Input: part model. Units: mm. Frame: model coordinates. A direction names the side the tool comes from. Coordinates: 2 decimals unless noted, no trailing zeros. Loops run counter-clockwise (first coordinate to the right, second up) from the corner with the lowest first, then second, coordinate; pieces in that order, holes last.
(1) Section C-C, the plane y = 5.5. Return loops of the section in (x, z), then the cut area to 3 significant figures.
(2) Mould query, pull axis Z, two halves, no side actions, for faces 1 (the face through (43, 5, 80)), 2 (the face through (10, 5, 55)), 3 (the face through (13.01, 4.93, 97.15)). Classes: released by +Z, released by -Z, zero draft, split by the parting line, or undercut.
(3) Line query: L1, parallel to X at y = 27, z = 0; L2, parallel to X at y = 9, z = 38; L3, parallel to X at y = 24, z = -1. Output: solid intervals per line, ascending.
(4) Contact query for flat-ended pins moving along their axis: P1, Ø11, axis at y = 4.5, z = 47, coming from the -X side; P2, Ø3, axis at y = 21.5, z = 2, coming from the -X side; P3, Ø8, axis at x = 75.5, y = 19, coming from the -Z side. Output: stop coordinate, or through.
(5) Section B-B, the plane z = 0. Return loops of the section in (x, y), then the cut area to 3 significant figures.
(6) Section D-D, the plane z = 62. Return loops of the section in (x, y).
(7) Section A-A, the plane x = 47. Return loops of the section in (y, z), then the cut area to 3 significant figures.
(8) Set-up query: faces 4 (the face through (-19.524, 24.164, -4.336)), 5 (the face through (40, 10, 59)), 6 (the face through (70, 5, 55)). Return all of +Z, -Z, +X, -X, +Y, -Y with unobstructed straight access to the full face (end or side cutting, diameter ignored); none if empty.
```python
from build123d import *

# Parameters (mm, degrees)
SKETCH1_R           = 20
BOSS_EXTRUDE1_DEPTH = 40
SKETCH2_R           = 10
CUT_EXTRUDE1_DEPTH  = 49.989794856
SKETCH3_R           = 20
BOSS_EXTRUDE2_DEPTH = 30
SKETCH4_R           = 10
CUT_EXTRUDE2_DEPTH  = 107.301458127
SKETCH5_W           = 80
SKETCH5_H           = 10
BOSS_EXTRUDE3_DEPTH = 30
BOSS_EXTRUDE4_DEPTH = 10
BOSS_EXTRUDE5_DEPTH = 10


with BuildPart() as part:
    # Sketch1 → Boss-Extrude1 (new body)
    with BuildSketch(Plane(origin=(0, 0, 0), x_dir=(1, 0, 0), z_dir=(0, 1, 0))):
        with Locations(Location((0, 0, 0), (0, 0, 270))):
            Circle(SKETCH1_R)
    extrude(amount=BOSS_EXTRUDE1_DEPTH)

    # Sketch2 → Cut-Extrude1 (cut, through all)
    with BuildSketch(Plane(origin=(0, 40, 0), x_dir=(1, 0, 0), z_dir=(0, 1, 0))):
        with Locations(Location((0, 0, 0), (0, 0, 270))):
            Circle(SKETCH2_R)
    extrude(amount=-CUT_EXTRUDE1_DEPTH, mode=Mode.SUBTRACT)



with BuildPart() as body_2:
    # Sketch3 → Boss-Extrude2 (new body)
    with BuildSketch(Plane(origin=(0, 0, 0), x_dir=(1, 0, 0), z_dir=(0, 1, 0))):
        with Locations(Location((80, 0, 0), (0, 0, 270))):
            Circle(SKETCH3_R)
    extrude(amount=BOSS_EXTRUDE2_DEPTH)

    # Sketch4 → Cut-Extrude2 (cut, through all)
    with BuildSketch(Plane(origin=(0, 30, 0), x_dir=(1, 0, 0), z_dir=(0, 1, 0))):
        with Locations(Location((80, 0, 0), (0, 0, 270))):
            Circle(SKETCH4_R)
    extrude(amount=-CUT_EXTRUDE2_DEPTH, mode=Mode.SUBTRACT)


with BuildPart() as part_1:
    add(part.part)

    add(body_2.part)  # Boss-Extrude3 merges body 2
    # Sketch5 → Boss-Extrude3 (add)
    with BuildSketch(Plane(origin=(0, 30, 0), x_dir=(1, 0, 0), z_dir=(0, 1, 0))):
        with Locations((40, -15)):
            Rectangle(SKETCH5_W, SKETCH5_H)
    extrude(amount=-BOSS_EXTRUDE3_DEPTH)

    # Sketch6 → Boss-Extrude4 (add)
    with BuildSketch(Plane.XZ):
        with BuildLine():
            Line((0, 20), (80, 20))
            ThreePointArc((80, 20), (100, 0), (80, -20))
            Line((80, -20), (0, -20))
            ThreePointArc((0, -20), (-20, 0), (0, 20))
        make_face()
    extrude(amount=-BOSS_EXTRUDE4_DEPTH)

    # Sketch7 → Boss-Extrude5 (add)
    with BuildSketch(Plane(origin=(0, 0, 0), x_dir=(1, 0, 0), z_dir=(0, 1, 0))):
        with BuildLine():
            Line((10, -20), (70, -20))
            Line((70, -20), (70, -90))
            ThreePointArc((70, -90), (67.071067812, -97.071067812), (60, -100))
            Line((60, -100), (20, -100))
            ThreePointArc((20, -100), (12.928932188, -97.071067812), (10, -90))
            Line((10, -90), (10, -20))
        make_face()
        with BuildLine():
            Line((35, -60), (50, -60))
            ThreePointArc((50, -60), (60, -70), (50, -80))
            Line((50, -80), (35, -80))
            ThreePointArc((35, -80), (25, -70), (35, -60))
        make_face(mode=Mode.SUBTRACT)
    extrude(amount=BOSS_EXTRUDE5_DEPTH)


solid = part_1.part
```
Report:
1. outline: (0, -20) - (80, -20) arc R20 ccw to (80, 20) - (70, 20) - (70, 90) arc R10 ccw to (60, 100) - (20, 100) arc R10 ccw to (10, 90) - (10, 20) - (0, 20) arc R20 ccw to start; hole (35, 60) - (50, 60) arc R10 ccw to (50, 80) - (35, 80) arc R10 ccw to start
1. area: 8,600 mm2
2. face 1: undercut
2. face 2: zero draft
2. face 3: released by +Z
3. L1: x = -20 to -10, 10 to 20, 60 to 70, 90 to 100
3. L2: x = 10 to 70
3. L3: x = -19.97 to -9.95, 9.95 to 19.97, 60.03 to 70.05, 89.95 to 99.97
4. P1: stops at x = 10
4. P2: stops at x = -19.99
4. P3: stops at z = -19.99
5. outline: (-20, 0) - (100, 0) - (100, 30) - (90, 30) - (90, 10) - (70, 10) - (70, 30) - (60, 30) - (60, 10) - (20, 10) - (20, 40) - (10, 40) - (10, 10) - (-10, 10) - (-10, 40) - (-20, 40) - close
5. area: 2,200 mm2
6. outline: (10, 0) - (29, 0) - (29, 10) - (10, 10) - close; (56, 0) - (70, 0) - (70, 10) - (56, 10) - close
7. outline: (0, -20) - (10, -20) - (10, 10) - (30, 10) - (30, 20) - (10, 20) - (10, 60) - (0, 60) - close; (0, 80) - (10, 80) - (10, 100) - (0, 100) - close
7. area: 1,200 mm2
8. face 4: +Y
8. face 5: +Z, +X, -X, +Y
8. face 6: +Z, +X, +Y, -Y
